Design review of the part built by this model. Coordinates are the model's own, in mm. Face numbers are marked on the shaded views. A direction names the side the tool comes from. Give positions to 0.01 mm unless a question says otherwise; leave off trailing zeros. Loops run counter-clockwise (first coordinate to the right, second up) from the corner with the lowest first, then second, coordinate; pieces in that order, holes last. Notation, with made-up numbers: (52.25, 42.5) -> (99.25, 42.5) arc R26 cw to (99.25, 76.5) -> close; hole circle Ø7 at (-15, 70.5). An arc over 180 degrees is marked (long way). Answer as CSV lines item,"result".
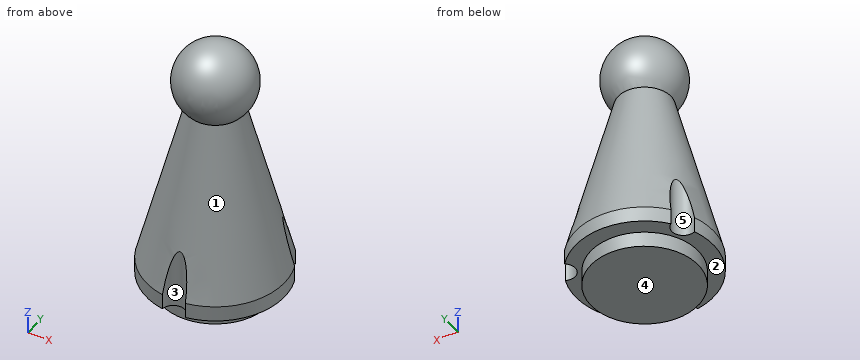
from build123d import *

# Parameters (mm, degrees)
F0_R      = 7
F1_DEPTH  = 2
F2_R      = 9
F3_DEPTH  = 2
F3_FACE_R = 9
F5_R      = 2.5
F9_R      = 1.5
F10_DEPTH = 32.001


with BuildPart() as f1:
    # F0 (on Top) → F1 (new body)
    with BuildSketch(Plane.XY):
        Circle(F0_R)
    extrude(amount=F1_DEPTH)

    # F2 (on face) → F3 (join)
    with BuildSketch(Plane.XY.offset(2)):
        Circle(F2_R)
    extrude(amount=F3_DEPTH)

    # F3_face (on face) → F6 section 0
    with BuildSketch(Plane.XY.offset(4)):
        Circle(F3_FACE_R)
    # F5 (on offset) → F6 section 1
    with BuildSketch(Plane.XY.offset(29)):
        Circle(F5_R)
    loft()

    # F7 (on face) → F8 (revolve)
    with BuildSketch(Plane.XY.offset(29)):
        with BuildLine():
            ThreePointArc((-5, 0), (0, -5), (5, 0))
            Line((5, 0), (2.5, 0))
            ThreePointArc((2.5, 0), (0, -2.5), (-2.5, 0))
            Line((-2.5, 0), (-5, 0))
        make_face()
        with BuildLine():
            Line((-2.5, 0), (2.5, 0))
            ThreePointArc((2.5, 0), (0, 2.5), (-2.5, 0))
        make_face()
    revolve(axis=Axis((0, 0, 29), (1, 0, 0)))

    # F9 (on face) → F10 (cut, through all)
    with BuildSketch(Plane(origin=(0, 0, 2), x_dir=(1, 0, 0), z_dir=(0, 0, -1))):
        with Locations((0, 9)):
            Circle(F9_R)
        with Locations((-7.7942286341, -4.5)):
            Circle(F9_R)
        with Locations((7.7942286341, -4.5)):
            Circle(F9_R)
    extrude(amount=-F10_DEPTH, mode=Mode.SUBTRACT)


solid = f1.part
Q1. We need section C-C, the plane z = 21. State the section outline as (x, y) points, and give its area (3 significant figures).
Filled sheet:
outline,"circle Ø9.16 at (0, 0)"
area,"65.9 mm^2"
Q2. We need section A-A, the plane z = 24.5. State the section outline as (x, y) points.
Filled sheet:
outline,"circle Ø7.34 at (0, 0)"
Q3. Clearance check with flat-ended pins moving along their axes: pin 1 Ø1 at (y, z) = (5.5, 5) entering from -X; pin 2 Ø10 at (x, z) = (-4.5, 24) entering from -Y; pin 3 Ø4 at (x, z) = (0, 14) entering from -Y. State where each tip first meets the part, or that it passes through.
Filled sheet:
pin 1,"stops at x = -6.83"
pin 2,"stops at y = -4.69"
pin 3,"stops at y = -6.92"
Q4. We need section B-B, the plane x = 0. State the section outline as (y, z) points, and give its area (3 significant figures).
Filled sheet:
outline,"(-7.5, 2) -> (-7, 2) -> (-7, 0) -> (7, 0) -> (7, 2) -> (9, 2) -> (9, 4) -> (3.44, 25.37) arc R5 ccw (long way) to (-3.44, 25.37) -> (-7.5, 9.77) -> close"
area,"395 mm^2"
Q5. For the marked faces 1 and 2, list the 3-axis set-ups (+Z, -Z, +X, -X, +Y, -Y) from which the entire face can be reached by the end or side of a thin tool; tool diameter is ignored.
Filled sheet:
face 1,"none"
face 2,"-Z"
Q6. We need section D-D, the plane z = 8. State the section outline as (x, y) points.
Filled sheet:
outline,"(-7.34, 3.07) arc R7.96 ccw to (-1.01, -7.9) arc R1.5 cw to (1.01, -7.9) arc R7.96 ccw to (7.34, 3.07) arc R1.5 cw to (6.33, 4.83) arc R7.96 ccw to (-6.33, 4.83) arc R1.5 cw to start"
Q7. The part is to be moulded in two halves that separate along Y. For the marked faces 3, 4 and 5, say which applies: pulls with the +Y half, pulls with the -Y half, needs draft (parallel to the pull), parting line crosses it, or undercut.
Filled sheet:
face 3,"pulls with the -Y half"
face 4,"needs draft"
face 5,"undercut"
